Check sheet for the modelled part. Datum: model origin and axes. Units: mm. A direction names the side the tool comes from. Round coordinates to 2 decimals unless told otherwise and drop trailing zeros. Loops run counter-clockwise (first coordinate to the right, second up) from the corner with the lowest first, then second, coordinate; pieces in that order, holes last. Notation, with made-up numbers: M 74,57 L 85,57 A22 cw 85,91 Z; hole C 26.5,-29.5 d2. An arc over 180 degrees is marked long. One line per question, with ' | ' between items. Start each with the question number.
(1) Section check A-A (z = 1.05). Record the boundary of the cut face in (x, y), and give its area (3 significant figures).
(2) Tool access check on faces 4 (the face through (-92.68, -31.74, 1.57)), 5 (the face through (-116.29, -126.55, 1.57)), 6 (the face through (-112.803, -21.622, 1.565)). Record the directions out of +Z, -Z, +X, -X, +Y, -Y that give a thin tool (end or side, any length) a straight path to the whole face; none if there is none.
(3) Thickness scan on probe 1 along X at (y, z) = (-8.5, 1.05); probe 2 along Y at (x, z) = (-70, 1.45); probe 3 along X at (y, z) = (-15, 2.5). Record the ranges inside material, lowest first. Write a range as [from, to].
(4) Section check D-D (x = -35). Record the boundary of the cut face in (y, z) (3 decimals).
(5) Go/stop test with flat-tipped pins: P1, Ø10, axis at x = -16.5, y = 1, coming from the -Z side; P2, Ø1.6, axis at x = -44.5, z = 1, coming from the -Y side. Record where each tip stops, or that it passes through.
(6) Section check B-B (x = -101). Record the boundary of the cut face in (y, z) (3 decimals).
(7) Draft check along Y on faces 1 (the face through (-95, -33, 3.175)), 2 (the face through (-147.46, -57.59, 1.57)), 3 (the face through (-147.203, 12.979, 1.565)). Enter one of: +Y half, -Y half, draft (parallel to the pull), parting line (faces both ways), or undercut.
(8) Section check C-C (y = 9). Record the boundary of the cut face in (x, z) (3 decimals), and give its area (3 significant figures).
```python
from build123d import *

# Parameters (mm, degrees)
SKETCH1_R           = 6.35
BOSS_EXTRUDE1_DEPTH = 3.175


with BuildPart() as part:
    # Sketch1 → Boss-Extrude1 (new body)
    with BuildSketch(Plane.XY):
        with BuildLine():
            Line((-141.234566003, -128.730482523), (-90.62787534, -124.302970792))
            Line((-90.62787534, -124.302970792), (-97.468846126, -46.110316899))
            ThreePointArc((-97.468846126, -46.110316899), (-92.536470394, -31.580006545), (-78.491337127, -25.4))
            Line((-78.491337127, -25.4), (0, -25.4))
            Line((0, -25.4), (0, 25.4))
            Line((0, 25.4), (-140.859617964, 25.4))
            ThreePointArc((-140.859617964, 25.4), (-150.223040141, 21.279995637), (-153.511290629, 11.593122067))
            Line((-153.511290629, 11.593122067), (-141.234566003, -128.730482523))
        make_face()
        with Locations((-140.859617964, 12.7)):
            Circle(SKETCH1_R, mode=Mode.SUBTRACT)
        with BuildLine():
            Line((-103.570761891, -30.081711089), (-122.297606246, -12.921719815))
            ThreePointArc((-122.297606246, -12.921719815), (-122.689319517, -3.950010908), (-113.717610609, -3.558297638))
            Line((-113.717610609, -3.558297638), (-94.990766254, -20.718288911))
            ThreePointArc((-94.990766254, -20.718288911), (-94.599052984, -29.689997818), (-103.570761891, -30.081711089))
        make_face(mode=Mode.SUBTRACT)
    extrude(amount=BOSS_EXTRUDE1_DEPTH)


solid = part.part
```
The answers:
1) outline: M -153.51,11.59 L -141.23,-128.73 L -90.63,-124.3 L -97.47,-46.11 A19.05 cw -78.49,-25.4 L 0,-25.4 L 0,25.4 L -140.86,25.4 A12.7 ccw Z; hole C -140.86,12.7 d12.7; hole M -122.3,-12.92 L -103.57,-30.08 A6.35 ccw -94.99,-20.72 L -113.72,-3.56 A6.35 ccw Z | area: 12,400 mm²
2) face 4: +Z, -Z, +X | face 5: +Z, -Z, +X, -Y | face 6: +Z, -Z
3) probe 1: [-151.75, -124.35], [-108.32, 0] | probe 2: [-25.4, 25.4] | probe 3: [-151.18, -120.03], [-101.23, 0]
4) outline: M -25.4,0 L 25.4,0 L 25.4,3.175 L -25.4,3.175 Z
5) P1: z = 0 | P2: y = -25.4
6) outline: M -125.21,0 L -31.513,0 L -31.513,3.175 L -125.21,3.175 Z; M -15.212,0 L 25.4,0 L 25.4,3.175 L -15.212,3.175 Z
7) face 1: draft | face 2: -Y half | face 3: undercut
8) outline: M -153.284,0 L -146.02,0 L -146.02,3.175 L -153.284,3.175 Z; M -135.699,0 L 0,0 L 0,3.175 L -135.699,3.175 Z | area: 454 mm²
